from build123d import *

# Parameters (mm, degrees)
SKETCH_W  = 40
SKETCH_H  = 40
SKETCH_R  = 2.25
PAD_DEPTH = 5


with BuildPart() as part:
    # Sketch → Pad (new body)
    with BuildSketch(Plane.XY):
        Rectangle(SKETCH_W, SKETCH_H)
        with Locations((0, 13.75)):
            Circle(SKETCH_R, mode=Mode.SUBTRACT)
        with Locations((0, -13.75)):
            Circle(SKETCH_R, mode=Mode.SUBTRACT)
        with BuildLine():
            ThreePointArc((-4.999996, 5.15), (-10.149996, 2e-06), (-5, -5.15))
            Line((-5, -5.15), (5, -5.15))
            ThreePointArc((5, -5.15), (10.149996, 0), (4.999999, 5.15))
            Line((-4.999996, 5.15), (4.999999, 5.15))
        make_face(mode=Mode.SUBTRACT)
    extrude(amount=PAD_DEPTH)


solid = part.part
Could you check a few things on this model? Use its own coordinates, in mm. A direction names the side the tool comes from. Give positions to 0.01 mm unless a question says otherwise; leave off trailing zeros. Write each loop counter-clockwise with the first axis right and the second up, starting at its lowest first coordinate (ties: lowest second). Pieces come first, ordered by that corner, then holes. Notation, with made-up numbers: (-25, -27) - (4, -27) arc R14 cw to (4, -8) - close; hole circle Ø1 at (87, -18). An arc over 180 degrees is marked (long way). Use CSV: the item, a comma, the result in double quotes. Start each with the question number.
Item 1: I want a section at C-C, the plane z = 1.4. Please give me the cut outline in (x, y), then the cut area to 3 significant figures.
Item 2: I want a section at B-B, the plane x = 0. Please give me the cut outline in (y, z).
Item 3: If we mould it in two halves opening along Y, with no side actions, what happens to faces 3 (the face through (20, 0, 2)), 4 (the face through (10.15, -0.11, 2.46)), 5 (the face through (0, -20, 2))? For each: pulls with the +Y half, pulls with the -Y half, needs draft (parallel to the pull), parting line crosses it, or undercut.
Item 4: If I drill on line 1 along Y through (x, z) = (0, 1.6); line 2 along Y through (x, z) = (-4, 2.6); line 3 along Y through (x, z) = (1, 2.1), over which ranges is the centre line in solid material (lowest first)?
Item 5: For faces 1 (the face through (0, 9, 5)), 2 (the face through (0, 5.15, 2)), which set-ups out of +Z, -Z, +X, -X, +Y, -Y let a thin tool reach every point of the face, with its end or its side?
Item 6: I want a section at A-A, the plane y = 0. Please give me the cut outline in (x, z).
Item 7: I want a section at D-D, the plane x = 7. Please give me the cut outline in (y, z).
Findings:
1,outline,"(-20, -20) - (20, -20) - (20, 20) - (-20, 20) - close; hole (-5, -5.15) - (5, -5.15) arc R5.15 ccw to (5, 5.15) - (-5, 5.15) arc R5.15 ccw to start; hole circle Ø4.5 at (0, -13.75); hole circle Ø4.5 at (0, 13.75)"
1,area,"1,380 mm2"
2,outline,"(-20, 0) - (-16, 0) - (-16, 5) - (-20, 5) - close; (-11.5, 0) - (-5.15, 0) - (-5.15, 5) - (-11.5, 5) - close; (5.15, 0) - (11.5, 0) - (11.5, 5) - (5.15, 5) - close; (16, 0) - (20, 0) - (20, 5) - (16, 5) - close"
3,face 3,"needs draft"
3,face 4,"undercut"
3,face 5,"pulls with the -Y half"
4,line 1,"y = -20 to -16, -11.5 to -5.15, 5.15 to 11.5, 16 to 20"
4,line 2,"y = -20 to -5.15, 5.15 to 20"
4,line 3,"y = -20 to -15.77, -11.73 to -5.15, 5.15 to 11.73, 15.77 to 20"
5,face 1,"+Z, +X, -X, +Y, -Y"
5,face 2,"+Z, -Z"
6,outline,"(-20, 0) - (-10.15, 0) - (-10.15, 5) - (-20, 5) - close; (10.15, 0) - (20, 0) - (20, 5) - (10.15, 5) - close"
7,outline,"(-20, 0) - (-4.75, 0) - (-4.75, 5) - (-20, 5) - close; (4.75, 0) - (20, 0) - (20, 5) - (4.75, 5) - close"
